Geometry check sheet. Reference: drawing and pictorial views, mm from the part's lowest x, y, z. Round coordinates to 2 decimals unless told otherwise and drop trailing zeros. Write each loop counter-clockwise with the first axis right and the second up, starting at its lowest first coordinate (ties: lowest second). Pieces come first, ordered by that corner, then holes. Notation, with made-up numbers: (88, 74.5) -> (129, 74.5) arc R23 cw to (129, 99.5) -> close; hole circle Ø10 at (-12.5, 15). An arc over 180 degrees is marked (long way). Write item = value, one per line.
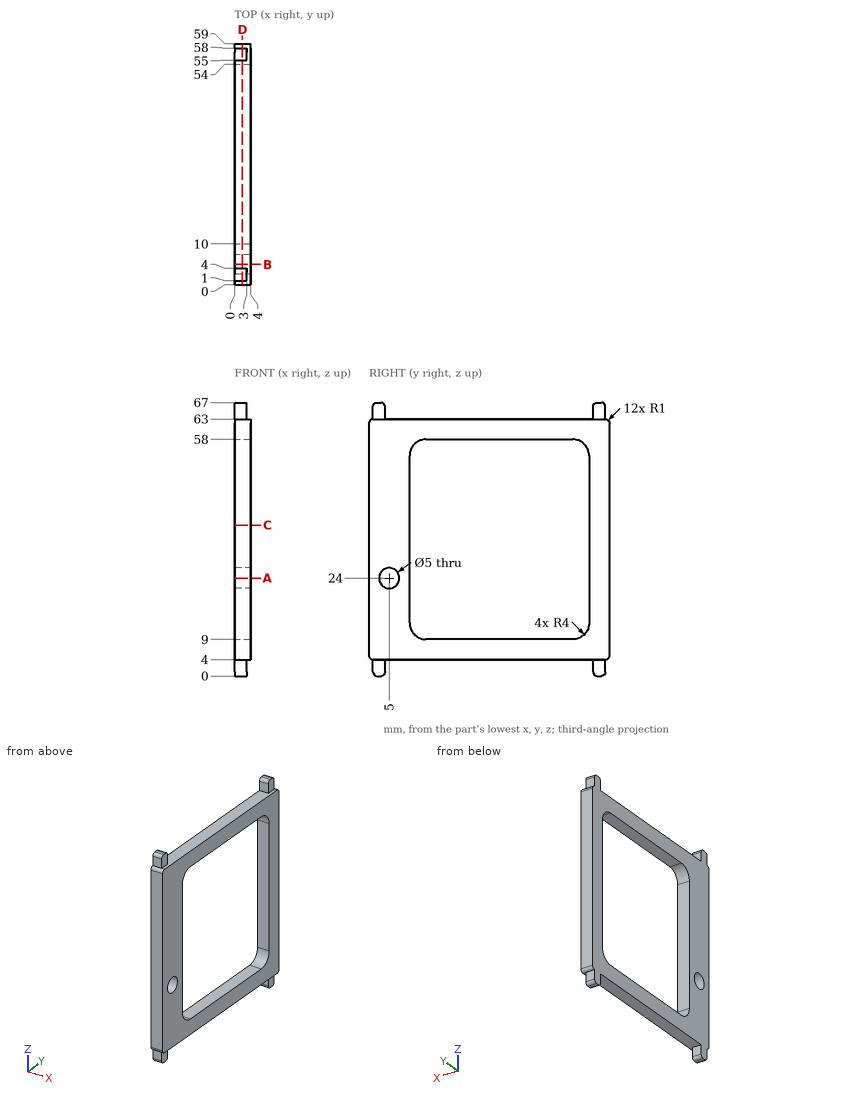
(1) Sectioned sample at A-A on z = 24. Enter the section's corners in (x, y).
Worked answers:
outline = (0, 0) -> (4, 0) -> (4, 2.5) -> (0, 2.5) -> close; (0, 7.5) -> (4, 7.5) -> (4, 10) -> (0, 10) -> close; (0, 54) -> (4, 54) -> (4, 59) -> (0, 59) -> close
(2) Sectioned sample at C-C on z = 37. Enter the section's corners in (x, y).
Worked answers:
outline = (0, 0) -> (4, 0) -> (4, 10) -> (0, 10) -> close; (0, 54) -> (4, 54) -> (4, 59) -> (0, 59) -> close
(3) Go/stop test with flat-tipped pins: P1, Ø0.9, axis at y = 56.5, z = 1.5, coming from the +X side; P2, Ø0.9, axis at x = 2, z = 2.5, coming from the +Y side; P3, Ø2, axis at x = 2.5, y = 23.5, coming from the +Z side; P4, Ø8, axis at y = 52, z = 39, coming from the -X side. Record where each tip stops, or that it passes through.
Worked answers:
P1 = 3
P2 = 58
P3 = 63
P4 = 0
(4) Sectioned sample at D-D on x = 1.9. Count the separate pieces of the cut face and the enclosed holes in it, then the cut area to 3 significant figures.
Worked answers:
separate_pieces = 1
enclosed_holes = 2
area = 1,360 mm²
(5) Material ranges on L1, parallel to Z at x = 1.9, y = 26; L2, parallel to Z at x = 1.8, y = 5; L3, parallel to Y at x = 3.2, z = 44.5, recorded low to high. Write a range as [from, to].
Worked answers:
L1 = [4, 9], [58, 63]
L2 = [4, 21.5], [26.5, 63]
L3 = [0, 10], [54, 59]
(6) Sectioned sample at B-B on y = 5. Enter the section's corners in (x, z), then the cut area to 3 significant figures.
Worked answers:
outline = (0, 4) -> (4, 4) -> (4, 21.5) -> (0, 21.5) -> close; (0, 26.5) -> (4, 26.5) -> (4, 63) -> (0, 63) -> close
area = 216 mm²
